Autodesk Fusion 360 part; units mm, degrees
cylinder "CylinderPrimitive1" add diameter 10 height 20 placed x (1, 0, 0) y (0, 1, 0) z (0, 0, 1) at (0, 0, 0)
chamfer "Chamfer1" distance 5 angle 45 1 edges at (-4.6616, -1.8081, 20)
component "Base" placed x (1, 0, 0) y (0, 1, 0) z (0, 0, 1) at (0, 0, 0)
Source: CAD feature listing. Evaluate the final solid. Frame: model axes, mm. Coordinates: 2 decimals unless noted, no trailing zeros. Loops run counter-clockwise (first coordinate to the right, second up) from the corner with the lowest first, then second, coordinate; pieces in that order, holes last. Notation, with made-up numbers: M -4,71 L 51,71 A19 ccw 51,90 Z; hole C -11.75,-32.5 d8. An arc over 180 degrees is marked long. Use a Markdown table: item, result. Add a question column.
Q1. First-contact query: pin 1 (5 mm diameter, centred on x = -2, z = 14.5, fed in from -Y); pin 2 (2 mm diameter, centred on x = -3.5, z = 11, fed in from -Y); pin 3 (2 mm diameter, centred on x = -2.5, y = -0.5, fed in from +Z); pin 4 (3 mm diameter, centred on x = -2.5, z = 8.5, fed in from +Y). Flat tips, straight axial feed; report the tip coordinate or a pass-through.
Q2. Section query B-B, the plane z = 6.5. Return loops of the section in (x, y), and give its area (3 significant figures).
Q3. Section query A-A, the plane z = 15.5. Return loops of the section in (x, y), and give its area (3 significant figures).
Q4. Material intervals for L1, parallel to Z at x = -3, y = -1.5; L2, parallel to Y at x = 1.5, z = 4.25; L3, parallel to Y at x = -0.75, z = 2, sorted ascending.
Result:
| question | item | result |
|---|---|---|
| 1 | pin 1 | stops at y = -5 |
| 1 | pin 2 | stops at y = -4.33 |
| 1 | pin 3 | stops at z = 18.45 |
| 1 | pin 4 | stops at y = 4.9 |
| 2 | outline | C 0,0 d10 |
| 2 | area | 78.5 mm2 |
| 3 | outline | C 0,0 d9 |
| 3 | area | 63.6 mm2 |
| 4 | L1 | z = 0 to 16.65 |
| 4 | L2 | y = -4.77 to 4.77 |
| 4 | L3 | y = -4.94 to 4.94 |
